Check sheet for the modelled part. Datum: model origin and axes. Units: mm. A direction names the side the tool comes from. Give positions to 0.01 mm unless a question says otherwise; leave off trailing zeros. Loops run counter-clockwise (first coordinate to the right, second up) from the corner with the lowest first, then second, coordinate; pieces in that order, holes last. Notation, with made-up numbers: M 67,56 L 106,56 A32 cw 106,89 Z; hole C -2,50 d11. An arc over 180 degrees is marked long. Use one line per item in the form item = value.
Autodesk Inventor part; units mm, degrees
ref_plane "YZ Plane" through (0, 0, 0) normal (1, 0, 0) x (0, 1, 0)
ref_plane "XZ Plane" through (0, 0, 0) normal (0, 1, 0) x (-1, 0, 0)
ref_plane "XY Plane" through (0, 0, 0) normal (0, 0, 1) x (1, 0, 0)
sketch "Sketch1" plane through (0, 0, 0) normal (0, 1, 0) x (-1, 0, 0)
  line L0 (7.074, 9.2769) -> (0.074, 9.2769)
  line L1 (0.074, 9.2769) -> (0.074, -2.7231)
  line L2 (0.074, -2.7231) -> (7.074, -2.7231)
  line L3 (7.074, -2.7231) -> (7.074, 9.2769)
  line L4 (5.324, 6.2769) -> (1.824, 6.2769)
  line L5 (1.824, 6.2769) -> (1.824, 0.2769)
  line L6 (1.824, 0.2769) -> (5.324, 0.2769)
  line L7 (5.324, 0.2769) -> (5.324, 6.2769)
  point P0 (0, 0)
  dimension "d0" = 7
  dimension "d1" = 12
  dimension "d28" = 1.75
  dimension "d29" = 1.75
  dimension "d30" = 3
  dimension "d31" = 3
extrude "Extrusion1" add sketch "Sketch1" along normal blind 1
sketch "Sketch3" plane through (0, 1, 0) normal (0, 1, 0) x (1, 0, 0)
  circle A0 centre (-5.324, -8.0269) radius 0.375
  line L0 (-7.074, -9.2769) -> (-0.074, -9.2769)
  line L1 (-7.074, 2.7231) -> (-7.074, -9.2769)
  circle A1 centre (-1.824, -8.0269) radius 0.375
  circle A2 centre (-5.324, 1.4731) radius 0.375
  circle A3 centre (-1.824, 1.4731) radius 0.375
  point P0 (0, 0)
  dimension "d8" = 0.75
  dimension "d9" = 1.25
  dimension "d10" = 1.75
  dimension "d13" = 3.5
  dimension "d16" = 9.5
extrude "Extrusion3" cut sketch "Sketch3" against normal blind 5
sketch "Sketch7" plane through (0, 1, 0) normal (0, 1, 0) x (1, 0, 0)
  line L0 (-1.824, -6.2769) -> (-5.324, -6.2769)
  line L1 (-1.824, -0.2769) -> (-1.824, -6.2769)
  line L2 (-5.324, -6.2769) -> (-1.824, -6.2769)
  line L3 (-1.824, -6.2769) -> (-1.824, -0.2769)
  line L4 (-1.824, -0.2769) -> (-5.324, -0.2769)
  line L5 (-5.324, -0.2769) -> (-5.324, -6.2769)
  line L6 (-5.824, -6.7769) -> (-1.324, -6.7769)
  line L7 (-1.324, -6.7769) -> (-1.324, 0.2231)
  line L8 (-1.324, 0.2231) -> (-5.824, 0.2231)
  line L9 (-5.824, 0.2231) -> (-5.824, -6.7769)
  point P0 (0, 0)
  dimension "d32" = 0.5
extrude "Extrusion5" add sketch "Sketch7" along normal blind 5
sketch "Sketch8" plane through (-5.824, 1, 6.7769) normal (0, 0, 1) x (1, 0, 0)
  circle A0 centre (2.25, 2.625) radius 0.375
  line L0 (0, 5) -> (4.5, 5)
  line L1 (0, 0) -> (0, 5)
  point P0 (5.824, -1)
  dimension "d35" = 0.75
  dimension "d36" = 2
  dimension "d37" = 2.25
extrude "Extrusion6" cut sketch "Sketch8" against normal through all
properties part number "Lens Holder"
1) Release check for a two-part mould opening along Z. For faces 5 (the face through (-3.5, 0.5, -2.723)), 6 (the face through (-3.6, 0.5, 9.277)), 7 (the face through (-1.824, 3, 3)), 8 (the face through (-5.324, 3, 3)) record: pulls with the +Z half, pulls with the -Z half, needs draft (parallel to the pull), parting line crosses it, or undercut.
Evaluation:
face_5 = pulls with the -Z half
face_6 = pulls with the +Z half
face_7 = undercut
face_8 = undercut
2) Section check A-A (z = 2). Record the cut outline in (x, y), then the cut area to 3 significant figures.
Evaluation:
outline = M -7.07,0 L -5.32,0 L -5.32,6 L -5.82,6 L -5.82,1 L -7.07,1 Z; M -1.82,0 L -0.07,0 L -0.07,1 L -1.32,1 L -1.32,6 L -1.82,6 Z
area = 8.50 mm^2
3) Set-up check for faces 1 (the face through (-4, 3, 6.777)), 2 (the face through (-3, 3, -0.223)), 3 (the face through (-5.824, 3, 3)), 4 (the face through (-1.324, 3, 3)): record each of +Z, -Z, +X, -X, +Y, -Y from which the full face is reachable in a straight line by a thin tool's end or side.
Evaluation:
face_1 = +Z, +X, -X, +Y
face_2 = -Z, +X, -X, +Y
face_3 = +Z, -Z, -X, +Y
face_4 = +Z, -Z, +X, +Y
4) Scan lines: line 1 (X direction, y = 3.2, z = 0.75); line 2 (Z direction, x = -2.5, y = 1.8); line 3 (Y direction, x = -1.25, z = 8.5). Record each from-to range of solid material in increasing order.
Evaluation:
line_1 = -5.82 to -5.32, -1.82 to -1.32
line_2 = -0.22 to 0.28, 6.28 to 6.78
line_3 = 0 to 1
5) Section check B-B (y = 2.3). Record the cut outline in (x, z).
Evaluation:
outline = M -5.82,-0.22 L -1.32,-0.22 L -1.32,6.78 L -5.82,6.78 Z; hole M -5.32,0.28 L -1.82,0.28 L -1.82,6.28 L -5.32,6.28 Z
6) Section check D-D (y = 0.75). Record the cut outline in (x, z) (3 decimals), then the cut area to 3 significant figures.
Evaluation:
outline = M -7.074,-2.723 L -0.074,-2.723 L -0.074,9.277 L -7.074,9.277 Z; hole C -5.324,-1.473 d0.75; hole C -5.324,8.027 d0.75; hole M -5.324,0.277 L -1.824,0.277 L -1.824,6.277 L -5.324,6.277 Z; hole C -1.824,-1.473 d0.75; hole C -1.824,8.027 d0.75
area = 61.2 mm^2
7) Depth check by flat-ended pin: pin 1 Ø2 at (x, y) = (-4, 3.5) entering from -Z; pin 2 Ø2 at (x, y) = (-4, 3) entering from +Z; pin 3 Ø2.5 at (y, z) = (4, 2) entering from +X. Enter the tip coordinate at first touch or a pass-through.
Evaluation:
pin_1 = -0.22
pin_2 = 6.78
pin_3 = -1.32
8) Section check C-C (x = -4.5). Record the cut outline in (y, z).
Evaluation:
outline = M 0,-2.72 L 1,-2.72 L 1,-0.22 L 6,-0.22 L 6,0.28 L 0,0.28 Z; M 0,6.28 L 6,6.28 L 6,6.78 L 1,6.78 L 1,9.28 L 0,9.28 Z
